Can you work these out from the model? Positions are in its coordinate system, mm. A direction names the side the tool comes from. Coordinates: 2 decimals unless noted, no trailing zeros. Order: outer loops, then holes, each group sorted by start corner. A loop starts at its lowest first (then second) coordinate and runs counter-clockwise, first axis right, second up. Notation, with made-up numbers: (17, -4.5) -> (66, -4.5) arc R25 ccw to (66, 26.5) -> close; hole circle Ø4 at (14.25, -15.75). An arc over 180 degrees is marked (long way). Answer in a Markdown table with one row per item. Add a question column.
1. On a 3-axis mill with a long thin cutter (end or side, diameter ignored), from which of +Z, -Z, +X, -X, +Y, -Y can I reach the whole of each face in a straight line? I mean faces 1 (the face through (-62.086, 1.487, 26.536)), 2 (the face through (58.76, -7, 32)), 3 (the face through (-1, -35, 40.044)). Say none if no direction works.
2. Imagine slicing it at D-D on y = -17. Write out the boundary of the cut face in (x, z).
3. Imagine slicing it at C-C on x = 35. Write out the boundary of the cut face in (y, z), plus the area to 3 significant figures.
4. We'd pull the mould along Y, two halves only. Please class faces 4 (the face through (-1, -30.949, 25)), 5 (the face through (-1, -38.08, 24)), 6 (the face through (-1, 38.08, 24)), 7 (the face through (4.5, 31.2, 0)): pulls with the +Y half, pulls with the -Y half, needs draft (parallel to the pull), parting line crosses it, or undercut.
5. Will this pin go through, and if not, where does the flat tip stop? pin 1 (3.5 mm diameter, centred on x = 7.5, y = 33.5, fed in from +Z).
6. Imagine slicing it at A-A on z = 56. Write out the boundary of the cut face in (x, y), plus the area to 3 significant figures.
7. Imagine slicing it at B-B on y = 0. Write out the boundary of the cut face in (x, z), plus the area to 3 significant figures.
8. If I drill on line 1 along X through (y, z) = (21.5, 48); line 2 along Z through (x, y) = (61, 0); line 3 along Y through (x, z) = (27, 35.5), over which ranges is the centre line in solid material (lowest first)? Write a range as [from, to].
from build123d import *

# Parameters (mm, degrees)
F0_W     = 130.6402087212
F0_H     = 76.1592537165
F1_DEPTH = 63.5
F2_W     = 117.5191476941
F2_H     = 61.8972182274
F3_DEPTH = 63.5
F4_W     = 78.7710472941
F4_H     = 23.4558616281
F5_DEPTH = 101.6
F6_R     = 6.8576505009
F7_DEPTH = 152.4


with BuildPart() as f1:
    # F0 (on Top) → F1 (new body)
    with BuildSketch(Plane.XY):
        Rectangle(F0_W, F0_H)
    extrude(amount=F1_DEPTH)

    # F2 (on face) → F3 (cut)
    with BuildSketch(Plane.XY.offset(63.5)):
        Rectangle(F2_W, F2_H)
    extrude(amount=-F3_DEPTH, mode=Mode.SUBTRACT)

    # F4 (on face) → F5 (cut)
    with BuildSketch(Plane.XZ.offset(38.0796268582)):
        with Locations((0, 51.772069186)):
            Rectangle(F4_W, F4_H)
    extrude(amount=-F5_DEPTH, mode=Mode.SUBTRACT)

    # F6 (on face) → F7 (cut)
    with BuildSketch(Plane(origin=(-65.3201043606, 0, 0), x_dir=(0, -1, 0), z_dir=(-1, 0, 0))):
        with Locations((0, 33.230535686)):
            Circle(F6_R)
    extrude(amount=-F7_DEPTH, mode=Mode.SUBTRACT)


solid = f1.part
Answers follow:
| question | item | result |
|---|---|---|
| 1 | face 1 | +X, -X |
| 1 | face 2 | +Z, -Z |
| 1 | face 3 | +Z, +Y, -Y |
| 2 | outline | (-65.32, 0) -> (-58.76, 0) -> (-58.76, 63.5) -> (-65.32, 63.5) -> close; (58.76, 0) -> (65.32, 0) -> (65.32, 63.5) -> (58.76, 63.5) -> close |
| 3 | outline | (-38.08, 0) -> (-30.95, 0) -> (-30.95, 40.04) -> (-38.08, 40.04) -> close; (30.95, 0) -> (38.08, 0) -> (38.08, 40.04) -> (30.95, 40.04) -> close |
| 3 | area | 571 mm² |
| 4 | face 4 | undercut |
| 4 | face 5 | pulls with the -Y half |
| 4 | face 6 | pulls with the +Y half |
| 4 | face 7 | needs draft |
| 5 | pin 1 | stops at z = 40.04 |
| 6 | outline | (-65.32, -38.08) -> (-39.39, -38.08) -> (-39.39, -30.95) -> (-58.76, -30.95) -> (-58.76, 30.95) -> (-39.39, 30.95) -> (-39.39, 38.08) -> (-65.32, 38.08) -> close; (39.39, -38.08) -> (65.32, -38.08) -> (65.32, 38.08) -> (39.39, 38.08) -> (39.39, 30.95) -> (58.76, 30.95) -> (58.76, -30.95) -> (39.39, -30.95) -> close |
| 6 | area | 1,550 mm² |
| 7 | outline | (-65.32, 0) -> (-58.76, 0) -> (-58.76, 26.37) -> (-65.32, 26.37) -> close; (-65.32, 40.09) -> (-58.76, 40.09) -> (-58.76, 63.5) -> (-65.32, 63.5) -> close; (58.76, 0) -> (65.32, 0) -> (65.32, 26.37) -> (58.76, 26.37) -> close; (58.76, 40.09) -> (65.32, 40.09) -> (65.32, 63.5) -> (58.76, 63.5) -> close |
| 7 | area | 653 mm² |
| 8 | line 1 | x = [-65.32, -58.76], [58.76, 65.32] |
| 8 | line 2 | z = [0, 26.37], [40.09, 63.5] |
| 8 | line 3 | y = [-38.08, -30.95], [30.95, 38.08] |
